Can you work these out from the model? Positions are in its coordinate system, mm. A direction names the side the tool comes from. Coordinates: 2 decimals unless noted, no trailing zeros. Write each loop counter-clockwise with the first axis right and the second up, starting at its lowest first coordinate (ties: lowest second). Pieces come first, ordered by that corner, then holes.
```python
from build123d import *

# Parameters (mm, degrees)
F1_DEPTH = 914.4
F2_R     = 6.985
F3_DEPTH = 177.801
F4_R     = 3.175
F5_R     = 6.35


with BuildPart() as f1:
    # F0 (on Front) → F1 (new body)
    with BuildSketch(Plane.XZ):
        Polygon((82.55, 0), (-82.55, 0), (-82.55, 184.15), (-88.9, 184.15), (-88.9, -6.35), (88.9, -6.35), (88.9, 184.15), (82.55, 184.15), align=None)
    extrude(amount=-F1_DEPTH)

    # F2 (on face) → F3 (cut, through all)
    with BuildSketch(Plane.YZ.offset(88.9)):
        with Locations((50.8, 139.7)):
            Circle(F2_R)
        with Locations((152.4, 88.9)):
            Circle(F2_R)
        with Locations((457.2, 139.7)):
            Circle(F2_R)
        with Locations((50.8, 38.1)):
            Circle(F2_R)
        with Locations((457.2, 38.1)):
            Circle(F2_R)
        with Locations((762, 88.9)):
            Circle(F2_R)
        with Locations((863.6, 38.1)):
            Circle(F2_R)
        with Locations((863.6, 139.7)):
            Circle(F2_R)
    extrude(amount=-F3_DEPTH, mode=Mode.SUBTRACT)

    # F4
    f4_edges = [f1.edges().sort_by_distance(p)[0] for p in [
        (88.9, 457.2, -6.35),
        (-88.9, 457.2, -6.35),
        (-82.55, 457.2, 0),
        (82.55, 457.2, 0),
    ]]
    fillet(f4_edges, radius=F4_R)

    # F5
    f5_edges = [f1.edges().sort_by_distance(p)[0] for p in [
        (-85.725, 0, 184.15),
        (85.725, 0, 184.15),
        (85.725, 914.4, 184.15),
        (-85.725, 914.4, 184.15),
    ]]
    fillet(f5_edges, radius=F5_R)


solid = f1.part
```
1. If we section it at C-C, the plane x = 64.5: List the corners of the cut face in (y, z) for me, plus the area to 3 significant figures.
2. I'm going to push a flat-ended pin straight in: P1, Ø12, axis at x = 2, y = 393, coming from the +Z side. Where does the tip first touch, or does it pass through?
3. We'd pull the mould along X, two halves only. Please class faces 1 (the face through (-88.9, 451, 92)), 2 (the face through (0, 0, -3)), 3 (the face through (82.55, 451, 95)): released by +X, released by -X, zero draft, split by the parting line, or undercut.
4. If we section it at B-B, the plane y = 784: List the corners of the cut face in (x, z) for me (3 decimals), plus the area to 3 significant figures.
5. Which directions (+Z, -Z, +X, -X, +Y, -Y) give clear straight access to the entire face, cutting with the end or side of a thin tool? Please do faces 4 (the face through (-1, 451, -6.35)), 5 (the face through (-82.55, 451, 92)).
6. If I drill on L1, parallel to Z at x = -85, y = 863; L2, parallel to Y at x = 85, z = 88, over which ranges is the centre line in solid material (lowest first)?
7. If we section it at A-A, the plane z = 117: List the corners of the cut face in (x, y) for me, plus the area to 3 significant figures.
Answers:
1. outline: (0, -6.35) - (914.4, -6.35) - (914.4, 0) - (0, 0) - close
1. area: 5,810 mm2
2. P1: stops at z = 0
3. face 1: released by -X
3. face 2: zero draft
3. face 3: undercut
4. outline: (-88.9, -3.175) arc R3.175 ccw to (-85.725, -6.35) - (85.725, -6.35) arc R3.175 ccw to (88.9, -3.175) - (88.9, 184.15) - (82.55, 184.15) - (82.55, 3.175) arc R3.175 cw to (79.375, 0) - (-79.375, 0) arc R3.175 cw to (-82.55, 3.175) - (-82.55, 184.15) - (-88.9, 184.15) - close
4. area: 3,470 mm2
5. face 4: -Z, +X, -X, +Y, -Y
5. face 5: +Z, +Y, -Y
6. L1: z = -6.35 to 31.14, 45.06 to 132.74, 146.66 to 184.15
6. L2: y = 0 to 145.47, 159.33 to 755.07, 768.93 to 914.4
7. outline: (-88.9, 0) - (-82.55, 0) - (-82.55, 914.4) - (-88.9, 914.4) - close; (82.55, 0) - (88.9, 0) - (88.9, 914.4) - (82.55, 914.4) - close
7. area: 11,600 mm2
